Autodesk Inventor part; units mm, degrees
ref_plane "YZ Plane" through (0, 0, 0) normal (1, 0, 0) x (0, 1, 0)
ref_plane "XZ Plane" through (0, 0, 0) normal (0, 1, 0) x (-1, 0, 0)
ref_plane "XY Plane" through (0, 0, 0) normal (0, 0, 1) x (1, 0, 0)
sketch "Sketch1" plane through (0, 0, 0) normal (1, 0, 0) x (0, 1, 0)
  line L0 (3.175, -4.4901) -> (3.175, -71.7099)
  line L1 (0, -71.7099) -> (0, -4.4901)
  arc A0 (3.175, -4.4901) -> (0, -4.4901) centre (1.5875, 0) ccw
  circle A1 centre (1.5875, 0) radius 3.175
  circle A2 centre (1.5875, -76.2) radius 3.175
  arc A3 (0, -71.7099) -> (3.175, -71.7099) centre (1.5875, -76.2) ccw
  point P0 (0, 0)
  point P1 (0, -73.4504)
  dimension "d7" = 6.35
  dimension "d0" = 3.175
  dimension "d2" = 6.35
  dimension "d3" = 1.5875
  dimension "d6" = 1.5875
extrude "Extrusion1" add sketch "Sketch1" along normal blind 25.4 contours L0 A3 L1 A0 | A2
sketch "Sketch2" plane through (25.4, 0, 0) normal (1, 0, 0) x (0, 0, -1)
  circle A0 centre (76.4423, 1.5875) radius 3.175
  arc A1 (71.7099, 0) -> (71.7099, 3.175) centre (76.2, 1.5875) ccw
  point P0 (0, 0)
  dimension "d8" = 0
  dimension "d9" = 6.35
extrude "Extrusion2" cut sketch "Sketch2" against normal through all
properties part number "aimingrails" material "Aluminum 6061"
Model file for the job. Use its own axes, mm. A direction names the side the tool comes from. Coordinates: 2 decimals unless noted, no trailing zeros. Order: outer loops, then holes, each group sorted by start corner. A loop starts at its lowest first (then second) coordinate and runs counter-clockwise, first axis right, second up. Notation, with made-up numbers: (0.25, -27) -> (25.25, -27) arc R17 ccw to (25.25, -22) -> close; hole circle Ø9 at (-5.75, -16). An arc over 180 degrees is marked (long way). Return JSON: item names as keys, results as strings. Group by question number.
Item 1: Saw through at D-D on z = -58. Write the cut outline in (x, y) (3 decimals), then the cut area to 3 significant figures.
Item 2: Saw through at A-A on z = 0. Write the cut outline in (x, y).
Item 3: Pull direction Y, two halves, no side cores. Call faces 1 (the flat face through (13, 0, -39)), 2 (the cylindrical face through (12.52, 1.77, -80.96)), 3 (the cylindrical face through (12.5, 4.6, -1)), 4 (the cylindrical face through (12.88, 1.73, -73.27)): pulls with the +Y half, pulls with the -Y half, needs draft (parallel to the pull), parting line crosses it, or undercut.
Item 4: Saw through at B-B on z = -76.2. Write the cut outline in (x, y).
Item 5: Tool access for faces 5 (the flat face through (13, 3.175, -38)), 6 (the flat face through (25.4, 2, -35)): list every direction of +Z, -Z, +X, -X, +Y, -Y with a clear straight run to the whole face (end or side of a thin tool).
Item 6: Wall check: line 1 along Z through (x, y) = (14.5, 1); line 2 along Z through (x, y) = (5, 3.75); line 3 along Z through (x, y) = (14, 0.5). Give the ranges that are in metal, low to high. Write a range as [from, to].
Item 7: Flat gauge pins, fed straight in: P1, Ø12.5, axis at x = 7.5, z = -48, coming from the +Y side (3 decimals); P2, Ø7.5, axis at x = 11.5, z = -48, coming from the -Y side; P3, Ø5.5, axis at y = 1.59, z = -76.44, coming from the -X side; P4, Ø1, axis at x = 17, z = -4, coming from the +Y side. Where does each tip first touch, or does it go through?
Item 8: Saw through at C-C on x = 17.5. State how many separate pieces and enclosed holes the cut face has, then the cut area to 3 significant figures.
Values found:
{
 "1": {"outline": "(0, 0) -> (25.4, 0) -> (25.4, 3.175) -> (0, 3.175) -> close", "area": "80.6 mm2"},
 "2": {"outline": "(0, -3.17) -> (25.4, -3.17) -> (25.4, -1.59) -> (0, -1.59) -> close; (0, 4.76) -> (25.4, 4.76) -> (25.4, 6.35) -> (0, 6.35) -> close"},
 "3": {"face 1": "pulls with the -Y half", "face 2": "parting line crosses it", "face 3": "undercut", "face 4": "undercut"},
 "4": {"outline": "(0, -3.17) -> (25.4, -3.17) -> (25.4, -1.58) -> (0, -1.58) -> close; (0, 4.75) -> (25.4, 4.75) -> (25.4, 6.35) -> (0, 6.35) -> close"},
 "5": {"face 5": "+X, -X, +Y", "face 6": "+Z, -Z, +X, +Y, -Y"},
 "6": {"line 1": "z = [-80.93, -79.56], [-73.32, -3.12], [3.12, 4.73]", "line 2": "z = [-80.44, -78.77], [-74.12, -71.96], [-4.24, -2.32], [2.32, 4.24]", "line 3": "z = [-80.84, -79.43], [-73.46, -2.98], [2.98, 4.64]"},
 "7": {"P1": "stops at y = 3.175", "P2": "stops at y = 0", "P3": "passes through", "P4": "stops at y = 4.82"},
 "8": {"separate pieces": "1", "enclosed holes": "2", "area": "291 mm2"}
}
